from build123d import *

# Parameters (mm, degrees)
SKETCH1_R                  = 150
SKETCH1_R_2                = 125
BOSS_EXTRUDE1_DEPTH        = 20
SKETCH1_2_R                = 125
BOSS_EXTRUDE2_DEPTH        = 100
SKETCH2_R                  = 75
BOSS_EXTRUDE3_DEPTH        = 100
F_15_0_15_DIAMETER_HOLE1_D = 15
CIRPATTERN1_COUNT          = 4


with BuildPart() as part:
    # Sketch1 → Boss-Extrude1 (new body)
    with BuildSketch(Plane(origin=(0, 0, 0), x_dir=(1, 0, 0), z_dir=(0, 1, 0))):
        with Locations(Location((0, 0, 0), (0, 0, 270))):
            Circle(SKETCH1_R)
        with Locations(Location((0, 0, 0), (0, 0, 270))):
            Circle(SKETCH1_R_2, mode=Mode.SUBTRACT)
    extrude(amount=BOSS_EXTRUDE1_DEPTH)

    # Sketch1_2 → Boss-Extrude2 (add)
    with BuildSketch(Plane(origin=(0, 0, 0), x_dir=(1, 0, 0), z_dir=(0, 1, 0))):
        with Locations(Location((0, 0, 0), (0, 0, 270))):
            Circle(SKETCH1_2_R)
    extrude(amount=BOSS_EXTRUDE2_DEPTH)

    # Sketch2 → Boss-Extrude3 (add)
    with BuildSketch(Plane(origin=(0, 100, 0), x_dir=(1, 0, 0), z_dir=(0, 1, 0))):
        with Locations(Location((0, 0, 0), (0, 0, 270))):
            Circle(SKETCH2_R)
    extrude(amount=BOSS_EXTRUDE3_DEPTH)

    # 15.0 _15_ Diameter Hole1 (through all)
    with Locations(Plane(origin=(0, 20, 0), x_dir=(1, 0, 0), z_dir=(0, 1, 0))):
        with Locations((137.5, 0)):
            f_15_0_15_diameter_hole1 = Hole(F_15_0_15_DIAMETER_HOLE1_D / 2)

    # CirPattern1: 15.0 _15_ Diameter Hole1 ×4 about axis
    cirpattern1_axis = Axis((0, 0, 0), (0, 1, 0))
    for i in range(1, CIRPATTERN1_COUNT):
        add(f_15_0_15_diameter_hole1.rotate(cirpattern1_axis, i * 360 / CIRPATTERN1_COUNT), mode=Mode.SUBTRACT)


solid = part.part
Input: part model. Units: mm. Frame: model coordinates. A direction names the side the tool comes from. Coordinates: 2 decimals unless noted, no trailing zeros. Order: outer loops, then holes, each group sorted by start corner. A loop starts at its lowest first (then second) coordinate and runs counter-clockwise, first axis right, second up.
1. Cut plane D-D, the plane x = -137.5. Return loops of the section in (y, z), plus the area to 3 significant figures.
Checked values:
outline: (0, -59.95) - (20, -59.95) - (20, -7.5) - (0, -7.5) - close; (0, 7.5) - (20, 7.5) - (20, 59.95) - (0, 59.95) - close
area: 2,100 mm2
2. Cut plane A-A, the plane z = -137.5. Return loops of the section in (x, y), plus the area to 3 significant figures.
Checked values:
outline: (-59.95, 0) - (-7.5, 0) - (-7.5, 20) - (-59.95, 20) - close; (7.5, 0) - (59.95, 0) - (59.95, 20) - (7.5, 20) - close
area: 2,100 mm2
3. Contact query for flat-ended pins moving along their axis: P1, Ø8, axis at x = -68, y = 75, coming from the -Z side; P2, Ø2, axis at y = 27, z = -85, coming from the +X side; P3, Ø5, axis at y = 127, z = -4.5, coming from the +X side. Output: stop coordinate, or through.
Checked values:
P1: stops at z = -107.37
P2: stops at x = 92.57
P3: stops at x = 74.97
4. Draft query along Z for faces 3 (the cylindrical face through (-2.87, 9.86, 130.57)), 4 (the cylindrical face through (-91.273, 9.86, -119.035)), 5 (the flat face through (1, 200, -1)). Return one class per face: +Z half, -Z half, draft (parallel to the pull), parting line (faces both ways), or undercut.
Checked values:
face 3: undercut
face 4: parting line
face 5: draft
5. Cut plane B-B, the plane x = -106.5. Return loops of the section in (y, z).
Checked values:
outline: (0, -105.63) - (20, -105.63) - (20, -65.44) - (100, -65.44) - (100, 65.44) - (20, 65.44) - (20, 105.63) - (0, 105.63) - close
6. Ray query, line 1 along X through (y, z) = (177, 2); line 2 along Y through (x, z) = (-109.5, 89); line 3 along Y through (x, z) = (15.5, 76). Return the intervals inside material, ascending.
Checked values:
line 1: x = -74.97 to 74.97
line 2: y = 0 to 20
line 3: y = 0 to 100
7. Cut plane C-C, the plane y = 127. Return loops of the section in (x, z).
Checked values:
outline: circle Ø150 at (0, 0)
8. Access query for faces 1 (the cylindrical face through (-45.636, 149.3, -59.517)), 2 (the cylindrical face through (-130.57, 9.86, -2.87)). Directions: +Z, -Z, +X, -X, +Y, -Y. A direction counts if a zero-diameter tool reaches every point of the face in a straight line with its end or side. Return the directions, or none.
Checked values:
face 1: +Y
face 2: +Y, -Y
